```python
from build123d import *

# Parameters (mm, degrees)
F0_R      = 19.05
F1_DEPTH  = 148.2
F3_W      = 12.7
F3_H      = 3.175
F4_DEPTH  = 25.4
F6_W      = 101.6
F6_H      = 31.79568
F7_DEPTH  = 25.4
F8_R      = 5.08
F9_DEPTH  = 72
F10_R     = 3.81
F11_DEPTH = 152.4


with BuildPart() as f1:
    # F0 (on Right) → F1 (new body)
    with BuildSketch(Plane.YZ):
        Circle(F0_R)
    extrude(amount=-F1_DEPTH)

    # F3 (on Front) → F4 (join, symmetric)
    with BuildSketch(Plane.XZ):
        with Locations((-38.1, -1.5875)):
            Rectangle(F3_W, F3_H)
        with Locations((-38.1, 1.5875)):
            Rectangle(F3_W, F3_H)
    extrude(amount=F4_DEPTH, both=True)

    # F2 (on Front) → F5 (revolve, cut)
    with BuildSketch(Plane.XZ):
        with BuildLine():
            ThreePointArc((-8.89, -16.51), (-4.182231, -8.844527), (-2.54, 0))
            Line((-2.54, 0), (-8.89, 0))
            Line((-8.89, 0), (-8.89, -16.51))
        make_face()
        Polygon((-8.89, -16.51), (-8.89, 0), (-148.2, 0), (-148.2, -13.97), (-145.66, -13.97), (-145.66, -16.51), (-76.2, -16.51), align=None)
    revolve(axis=Axis((-78.545, 0, 0), (-1, 0, 0)), mode=Mode.SUBTRACT)

    # F6 (on Front) → F7 (cut, symmetric)
    with BuildSketch(Plane.XZ):
        Polygon((-177.8, 1.27), (-76.2, 1.27), (-76.2, 26.052563), (-178.992286, 26.052563), align=None)
        with Locations((-127, -17.16784)):
            Rectangle(F6_W, F6_H)
    extrude(amount=F7_DEPTH, both=True, mode=Mode.SUBTRACT)

    # F8 (on face) → F9 (join)
    with BuildSketch(Plane.YZ):
        Circle(F8_R)
    extrude(amount=F9_DEPTH)

    # F10 (on face) → F11 (cut)
    with BuildSketch(Plane.YZ.offset(72)):
        Circle(F10_R)
    extrude(amount=-F11_DEPTH, mode=Mode.SUBTRACT)


solid = f1.part
```
CAD build for the part. Positions are in the model's coordinates, mm. A direction names the side the tool comes from. Round coordinates to 2 decimals unless told otherwise and drop trailing zeros. Write each loop counter-clockwise with the first axis right and the second up, starting at its lowest first coordinate (ties: lowest second). Pieces come first, ordered by that corner, then holes. Notation, with made-up numbers: (76, -16.5) - (101, -16.5) arc R33 ccw to (101, 17.5) - close; hole circle Ø10 at (-18.75, 26.25). An arc over 180 degrees is marked (long way). Return JSON: item names as keys, results as strings. Group by question number.
Item 1: Band-saw the part on B-B on x = -54. List the corners of the cut face in (y, z).
Item 2: Band-saw the part on C-C on x = 25. List the corners of the cut face in (y, z), plus the area to 3 significant figures.
Item 3: Mould opens along Y. For faces 1 (the face through (-76.2, 0, 17)), 2 (the face through (-40.13, -15.12, -11.59)), 3 (the face through (35.11, -0.83, -3.72)), 4 (the face through (-38, 25.4, 0)) say: +Y half, -Y half, draft (parallel to the pull), parting line (faces both ways), or undercut.
Item 4: Band-saw the part on A-A on x = -127. List the corners of the cut face in (y, z).
Item 5: Flat gauge pins, fed straight in: pin 1 Ø1 at (x, y) = (25, 7) entering from -Z; pin 2 Ø5 at (y, z) = (-23, -1) entering from +X; pin 3 Ø7.5 at (x, y) = (-38.5, -20.5) entering from -Z; pin 4 Ø6 at (y, z) = (-5.5, -11) entering from -X. Where does each tip first touch, or does it go through?
Item 6: Probe probe 1 along Y at (x, z) = (-78, 0); probe 2 along Z at (x, y) = (20, 0). List the from-to ranges inside material, lowest first.
Item 7: 3-axis set-ups, long thin cutter, end or side, ignore diameter. For faces 5 (the face through (-113, 18, -1.27)), 6 (the face through (-113, 18, 1.27)), 7 (the face through (-38, 22, 3.175)): which of +Z, -Z, +X, -X, +Y, -Y reach the whole face in a straight line?
Resolved:
{
 "1": {"outline": "circle Ø38.1 at (0, 0); hole circle Ø33.02 at (0, 0)"},
 "2": {"outline": "circle Ø10.16 at (0, 0); hole circle Ø7.62 at (0, 0)", "area": "35.5 mm²"},
 "3": {"face 1": "draft", "face 2": "parting line", "face 3": "undercut", "face 4": "+Y half"},
 "4": {"outline": "(-19.01, -1.27) - (-16.46, -1.27) arc R16.51 cw to (-16.46, 1.27) - (-19.01, 1.27) arc R19.05 ccw to start; (16.46, -1.27) - (19.01, -1.27) arc R19.05 ccw to (19.01, 1.27) - (16.46, 1.27) arc R16.51 cw to start"},
 "5": {"pin 1": "passes through", "pin 2": "stops at x = -31.75", "pin 3": "stops at z = -9.07", "pin 4": "stops at x = -7.87"},
 "6": {"probe 1": "y = -19.05 to -16.51, 16.51 to 19.05", "probe 2": "z = -5.08 to -3.81, 3.81 to 5.08"},
 "7": {"face 5": "-Z, -X, +Y, -Y", "face 6": "+Z, -X, +Y, -Y", "face 7": "+Z, +X, -X, +Y"}
}
